For this review, take the finished solid that the model builds, in its own axes (mm). A direction names the side the tool comes from. Give positions to 0.01 mm unless a question says otherwise; leave off trailing zeros. Loops run counter-clockwise (first coordinate to the right, second up) from the corner with the lowest first, then second, coordinate; pieces in that order, holes last. Notation, with made-up numbers: (-14, -25.75) -> (-5, -25.75) arc R27 cw to (-5, -1.75) -> close; hole circle Ø3 at (60.25, 49.25). An arc over 180 degrees is marked (long way). Answer as CSV lines item,"result". Start each with the question number.
Item 1: Add section B-B on z = 0. State the section outline as (x, y) points.
Item 2: Add section C-C on y = 24.5. State the section outline as (x, z) points, plus the area to 3 significant figures.
Item 3: The part is to be moulded in two halves that separate along X. For faces 1 (the face through (23, 18, 1.861)), 2 (the face through (1, -20, 1)), say which applies: +X half, -X half, draft (parallel to the pull), parting line (faces both ways), or undercut.
Item 4: Clearance check with flat-ended pins moving along their axes: P1, Ø5, axis at y = 40.5, z = -20, coming from the +X side; P2, Ø13, axis at x = 1, z = 6, coming from the +Y side; P3, Ø12.5, axis at x = 21, y = 12.5, coming from the -Z side. State where each tip first meets the part, or that it passes through.
Item 5: Add section A-A on x = 0. State the section outline as (y, z) points, plus the area to 3 significant figures.
Item 6: Add section D-D on z = 22.5. State the section outline as (x, y) points, plus the area to 3 significant figures.
Item 7: For L1, parallel to Z at x = -18, y = 33.5; L2, parallel to Z at x = -3.5, y = 18; L3, parallel to X at y = 51, z = 0, list the stretches that pass through material, from the lowest coordinate up. Write a range as from..to.
Item 8: Machinability: for faces 3 (the face through (-10, 18, -26)), 4 (the face through (29.224, 54.23, -19.619)), which of the approach directions +Z, -Z, +X, -X, +Y, -Y give a long, thin tool a straight path to every point of the face, cutting with its end or side? Answer none if there is none.
```python
from build123d import *

# Parameters (mm, degrees)
SKETCH2_R               = 37.5
SKETCH2_R_2             = 35
BOSS_EXTRUDE2_DEPTH     = 37.3
BOSS_EXTRUDE3_START     = 20
SKETCH3_R               = 37.5
BOSS_EXTRUDE3_DEPTH     = 20
SKETCH4_R               = 37.5
SKETCH4_R_2             = 35
BOSS_EXTRUDE4_DEPTH     = 40
CUT_EXTRUDE2_DEPTH      = 60
CUT_EXTRUDE2_DEPTH_BACK = 60
SKETCH5_R               = 50


with BuildPart() as part:
    # Sketch2 → Boss-Extrude2 (new body)
    # profile 1 of 3: a face of its own
    with BuildSketch(Plane(origin=(0, 0, 0), x_dir=(1, 0, 0), z_dir=(0, 1, 0))):
        with Locations(Location((0, 0, 0), (0, 0, 270))):
            Circle(SKETCH2_R)
        Circle(SKETCH2_R_2, mode=Mode.SUBTRACT)
    # profile 2 of 3: a face of its own
    with BuildSketch(Plane(origin=(0, 0, 0), x_dir=(1, 0, 0), z_dir=(0, 1, 0))):
        with BuildLine():
            ThreePointArc((28.693735847, 20.041694617), (0, 35), (-28.693735847, 20.041694617))
            Line((-28.693735847, 20.041694617), (-10, 20.041694617))
            Line((-10, 20.041694617), (-10, 31.75))
            Line((-10, 31.75), (10, 31.75))
            Line((10, 31.75), (10, 20.041694617))
            Line((10, 20.041694617), (28.693735847, 20.041694617))
        make_face()
    # profile 3 of 3: a face of its own
    with BuildSketch(Plane(origin=(0, 0, 0), x_dir=(1, 0, 0), z_dir=(0, 1, 0))):
        with BuildLine():
            Line((-10, -1.861454278), (-34.950464775, -1.861454278))
            ThreePointArc((-34.950464775, -1.861454278), (-34.090270263, -7.928018251), (-32.18529571, -13.751608636))
            Line((-32.18529571, -13.751608636), (32.18529571, -13.751608636))
            ThreePointArc((32.18529571, -13.751608636), (34.090270263, -7.928018251), (34.950464775, -1.861454278))
            Line((34.950464775, -1.861454278), (10, -1.861454278))
            Line((10, -1.861454278), (10, -8.5))
            Line((10, -8.5), (-10, -8.5))
            Line((-10, -8.5), (-10, -1.861454278))
        make_face()
    extrude(amount=BOSS_EXTRUDE2_DEPTH)

    # Sketch3 → Boss-Extrude3 (add)
    with BuildSketch(Plane.XZ.offset(BOSS_EXTRUDE3_START)):
        with Locations(Location((0, 0, 0), (0, 0, 270))):
            Circle(SKETCH3_R)
    extrude(amount=-BOSS_EXTRUDE3_DEPTH)

    # Sketch4 → Boss-Extrude4 (add)
    with BuildSketch(Plane(origin=(0, 37.3, 0), x_dir=(1, 0, 0), z_dir=(0, 1, 0))):
        with Locations(Location((0, 0, 0), (0, 0, 90))):
            Circle(SKETCH4_R)
        with Locations(Location((0, 0, 0), (0, 0, 34.933118398))):
            Circle(SKETCH4_R_2, mode=Mode.SUBTRACT)
    extrude(amount=BOSS_EXTRUDE4_DEPTH)

    # Sketch5 → Cut-Extrude2 (cut, two sides: drawn at the far end of the back side and taken through both)
    with BuildSketch(Plane.XY.offset(-CUT_EXTRUDE2_DEPTH_BACK)):
        with Locations((0, 94.8)):
            Circle(SKETCH5_R)
    extrude(amount=CUT_EXTRUDE2_DEPTH + CUT_EXTRUDE2_DEPTH_BACK, mode=Mode.SUBTRACT)


solid = part.part
```
Computed values:
1,outline,"(-37.5, -20) -> (37.5, -20) -> (37.5, 61.73) arc R50 cw to (35, 59.09) -> (35, 0) -> (-35, 0) -> (-35, 59.09) arc R50 cw to (-37.5, 61.73) -> close"
2,outline,"circle Ø75 at (0, 0); hole (-34.95, 1.86) arc R35 ccw to (-28.69, -20.04) -> (-10, -20.04) -> (-10, -31.75) -> (10, -31.75) -> (10, -20.04) -> (28.69, -20.04) arc R35 ccw to (34.95, 1.86) -> (10, 1.86) -> (10, 8.5) -> (-10, 8.5) -> (-10, 1.86) -> close; hole (-32.19, 13.75) -> (32.19, 13.75) arc R35 ccw to start"
2,area,"1,610 mm²"
3,face 1,"undercut"
3,face 2,"draft"
4,P1,"x = 33.17"
4,P2,"y = 37.3"
4,P3,"z = -34.48"
5,outline,"(-20, -37.5) -> (44.8, -37.5) -> (44.8, -35) -> (37.3, -35) -> (37.3, -31.75) -> (0, -31.75) -> (0, 8.5) -> (37.3, 8.5) -> (37.3, 13.75) -> (0, 13.75) -> (0, 35) -> (44.8, 35) -> (44.8, 37.5) -> (-20, 37.5) -> close"
5,area,"2,040 mm²"
6,outline,"(-30, -20) -> (30, -20) -> (30, 54.8) arc R50 cw to (26.81, 52.6) -> (26.81, 0) -> (-26.81, 0) -> (-26.81, 52.6) arc R50 cw to (-30, 54.8) -> close"
6,area,"1,540 mm²"
7,L1,"-32.9..-20.04, 1.86..13.75, 30.02..32.9"
7,L2,"-37.34..-31.75, 8.5..13.75, 34.82..37.34"
7,L3,"-37.5..-35, 35..37.5"
8,face 3,"+Y"
8,face 4,"+Z, -Z, +Y"
